Source: CAD feature listing. Evaluate the final solid. Frame: model axes, mm. A direction names the side the tool comes from. Give positions to 0.01 mm unless a question says otherwise; leave off trailing zeros. Order: outer loops, then holes, each group sorted by start corner. A loop starts at its lowest first (then second) coordinate and runs counter-clockwise, first axis right, second up. Notation, with made-up numbers: (85.25, 68) - (103.25, 68) arc R19 cw to (103.25, 91) - close; hole circle Ø4 at (72, 58). An arc over 180 degrees is marked (long way). Use CSV: the item, a comma, the result in double quotes.
Autodesk Inventor part; units mm, degrees
ref_plane "YZ Plane" through (0, 0, 0) normal (1, 0, 0) x (0, 1, 0)
ref_plane "XZ Plane" through (0, 0, 0) normal (0, 1, 0) x (-1, 0, 0)
ref_plane "XY Plane" through (0, 0, 0) normal (0, 0, 1) x (1, 0, 0)
sketch "Sketch1" plane through (0, 0, 0) normal (0, 1, 0) x (-1, 0, 0)
  circle A0 centre (0, 0) radius 5
  dimension "d0" = 10
extrude "Extrusion1" add sketch "Sketch1" against normal blind 20
sketch "Sketch2" plane through (0, 0, 0) normal (1, 0, 0) x (0, 1, 0)
  line L0 (0, 0) -> (-8, 0)
  line L1 (-8, 0) -> (-8, 5)
  line L2 (-8, 5) -> (0, 5)
  line L3 (0, 5) -> (0, 0)
  line L4 (-8, 5) -> (0, 5)
  line L5 (0, 5) -> (0, 10)
  line L6 (0, 10) -> (-8, 10)
  line L7 (-8, 10) -> (-8, 5)
  line L8 (0, -5) -> (0, 5)
  line L9 (0, -5) -> (-8, -5)
  line L10 (-8, -5) -> (-8, -10)
  line L11 (-8, -10) -> (0, -10)
  line L12 (0, -10) -> (0, -5)
  dimension "d3" = 8
  dimension "d4" = 5
  dimension "d5" = 8
  dimension "d6" = 5
  dimension "d7" = 5
extrude "Extrusion2" add sketch "Sketch2" along normal mid plane 5 contours L12 L11 L10 L9 | L2 L7 L6 L5
sketch "Sketch3" plane through (-2.5, -8, 10) normal (0, 0, 1) x (1, 0, 0)
  line L0 (2.5, 0) -> (0, 0)
  line L1 (2.5, 8) -> (5, 8)
  line L2 (0, 0) -> (5, 0)
  line L3 (5, 0) -> (5, 8)
  line L4 (5, 8) -> (0, 8)
  line L5 (0, 8) -> (0, 0)
extrude "Extrusion3" add sketch "Sketch3" against normal blind 20
sketch "Sketch4" plane through (0, 0, 0) normal (0, 1, 0) x (1, 0, 0)
  circle A0 centre (0, 0) radius 2.5
  dimension "d12" = 5
extrude "Extrusion4" cut sketch "Sketch4" against normal through all
sketch "Sketch5" plane through (2.5, 0, -10) normal (0, 0, -1) x (-1, 0, 0)
  line L0 (2.5, 0) -> (2.5, -5)
  circle A0 centre (2.5, -5) radius 2.5
  line L1 (0, 0) -> (0, -20)
  dimension "d15" = 5
extrude "Extrusion5" cut sketch "Sketch5" against normal blind 10
thread "Thread1"
sketch "Sketch6" plane through (-2.5, -8, 10) normal (0, 0, 1) x (1, 0, 0)
  line L0 (0, 0) -> (5, 0)
  line L1 (5, 8) -> (5, 0)
  line L2 (0, 0) -> (5, 0)
  line L3 (5, 0) -> (5, 8)
  line L4 (5, 8) -> (0, 8)
  line L5 (0, 8) -> (0, 0)
  point P0 (2.5, 8)
extrude "Extrusion6" cut sketch "Sketch6" against normal blind 2
sketch "Sketch7" plane through (2.5, 0, -10) normal (0, 0, -1) x (-1, 0, 0)
  line L0 (5, -8) -> (5, 0)
  line L1 (0, 0) -> (5, 0)
  line L2 (5, 0) -> (5, -8)
  line L3 (5, -8) -> (0, -8)
  line L4 (0, -8) -> (0, 0)
  point P0 (2.5, 0)
extrude "Extrusion7" cut sketch "Sketch7" against normal blind 2
properties part number "azimuth_gear_in" material "Aluminum 6061"
Item 1: Section A-A on x = -2.25. Return the cut outline in (y, z).
Filled in:
outline,"(-20, -4.47) - (-8, -4.47) - (-8, -8) - (-6.09, -8) - (-6.09, -1.09) - (-20, -1.09) - close; (-20, 1.09) - (0, 1.09) - (0, 8) - (-8, 8) - (-8, 4.47) - (-20, 4.47) - close; (-3.91, -8) - (0, -8) - (0, -1.09) - (-3.91, -1.09) - close"
Item 2: Set-up query: faces 1 (the flat face through (-2.5, -4, 6)), 2 (the flat face through (-2.5, -2, -6)), 3 (the flat face through (2.5, -3, -6)). Return all of +Z, -Z, +X, -X, +Y, -Y with unobstructed straight access to the full face (end or side cutting, diameter ignored); none if empty.
Filled in:
face 1,"+Z, -X, +Y, -Y"
face 2,"-Z, -X, +Y, -Y"
face 3,"-Z, +X, +Y, -Y"
Item 3: Section C-C on y = -16.5. Return the cut outline in (x, z), then the cut area to 3 significant figures.
Filled in:
outline,"circle Ø10 at (0, 0); hole circle Ø5 at (0, 0)"
area,"58.9 mm2"
Item 4: Material intervals for line 1 (Z direction, x = 0, y = -10.75); line 2 (Z direction, x = -1, y = -17); line 3 (X direction, y = -17, z = -0.5), sorted ascending. Write a range as from..to.
Filled in:
line 1,"z = -5..-2.5, 2.5..5"
line 2,"z = -4.9..-2.29, 2.29..4.9"
line 3,"x = -4.97..-2.45, 2.45..4.97"
Item 5: First-contact query: pin 1 (1.1 mm diameter, centred on y = -5, z = 6, fed in from +X); pin 2 (1.8 mm diameter, centred on y = -2, z = -7, fed in from -X); pin 3 (1.5 mm diameter, centred on x = 1.5, y = -14, fed in from -Z). Flat tips, straight axial feed; report the tip coordinate or a pass-through.
Filled in:
pin 1,"stops at x = 2.5"
pin 2,"stops at x = -2.5"
pin 3,"stops at z = -4.94"
Item 6: Section D-D on z = 3. Return the cut outline in (x, y), then the cut area to 3 significant figures.
Filled in:
outline,"(-4, -20) - (4, -20) - (4, 0) - (-4, 0) - close"
area,"160 mm2"
